```python
from build123d import *

# Parameters (mm, degrees)
BOSS_EXTRUDE2_DEPTH = 5
CHAMFER1_SIZE       = 0.7
FILLET1_R           = 2


with BuildPart() as part:
    # Sketch3 → Revolve1 (revolve)
    with BuildSketch(Plane.XY, mode=Mode.PRIVATE) as revolve1_sk:
        with BuildLine():
            Line((-41.25, 0), (-42.75, 0))
            Line((-42.75, 0), (-42.75, 15))
            Line((-42.75, 15), (-45, 15))
            add(Edge.make_bspline(
                [(-45, 15), (-45, 33.63701026), (-37.623115354, 59.484821268), (-12.301870518, 76.047426191), (0, 76.047426191)],
                knots=[0, 0, 0, 0, 0.584889903, 1, 1, 1, 1], degree=3))
            Line((0, 76.047426191), (0, 74.547426191))
            add(Edge.make_bspline(
                [(-43.490429879, 16.5), (-43.47825423, 17.447352), (-43.4296633, 19.355844405), (-43.235850844, 23.056930634), (-42.807900532, 27.545595426), (-41.986633297, 32.689505156), (-40.466663576, 39.238041503), (-37.743043327, 46.847747671), (-33.842433939, 53.728397249), (-29.961040028, 58.81673956), (-25.547541887, 63.646152056), (-20.393205683, 67.904061547), (-14.619902999, 71.183472612), (-10.010485444, 73.05966314), (-5.95200064, 74.059562605), (-2.594649158, 74.475411437), (-0.861029569, 74.547426191), (0, 74.547426191)],
                knots=[0.015975596, 0.015975596, 0.015975596, 0.015975596, 0.046726359, 0.077477122, 0.138978647, 0.200480172, 0.261981697, 0.384984748, 0.507987798, 0.569489323, 0.630990849, 0.753993899, 0.815495424, 0.87699695, 0.938498475, 0.969249237, 1, 1, 1, 1], degree=3))
            Line((-43.490429879, 16.5), (-42.75, 16.5))
            Line((-42.75, 16.5), (-41.25, 16.5))
            Line((-41.25, 16.5), (-41.25, 15))
            Line((-41.25, 15), (-41.25, 0))
        make_face()
    revolve(revolve1_sk.sketch.rotate(Axis((0, 0, 0), (0, 1, 0)), 270), axis=Axis((0, 0, 0), (0, 1, 0)))

    # Sketch4 → Boss-Extrude2 (add)
    with BuildSketch(Plane.XZ):
        with BuildLine():
            Line((-41.055602541, 4), (-4, 4))
            Line((-4, 4), (-4, 41.055602541))
            ThreePointArc((-4, 41.055602541), (0, 41.25), (4, 41.055602541))
            Line((4, 41.055602541), (4, 4))
            Line((4, 4), (41.055602541, 4))
            ThreePointArc((41.055602541, 4), (41.25, 0), (41.055602541, -4))
            Line((41.055602541, -4), (4, -4))
            Line((4, -4), (4, -41.055602541))
            ThreePointArc((4, -41.055602541), (0, -41.25), (-4, -41.055602541))
            Line((-4, -41.055602541), (-4, -4))
            Line((-4, -4), (-41.055602541, -4))
            ThreePointArc((-41.055602541, -4), (-41.25, 0), (-41.055602541, 4))
        make_face()
    extrude(amount=-BOSS_EXTRUDE2_DEPTH)

    # Chamfer1
    chamfer1_edges = [part.edges().sort_by_distance(p)[0] for p in [
        (0, 0, 42.75),
    ]]
    chamfer(chamfer1_edges, length=CHAMFER1_SIZE)

    # Fillet1
    fillet1_edges = [part.edges().sort_by_distance(p)[0] for p in [
        (-22.52780127, 5, 4),
        (-4, 5, 22.52780127),
        (4, 5, 22.52780127),
        (22.52780127, 5, 4),
        (22.52780127, 5, -4),
        (4, 5, -22.52780127),
        (-4, 5, -22.52780127),
        (-22.52780127, 5, -4),
        (-22.52780127, 0, -4),
        (-4, 0, -22.52780127),
        (4, 0, -22.52780127),
        (22.52780127, 0, -4),
        (22.52780127, 0, 4),
        (4, 0, 22.52780127),
        (-4, 0, 22.52780127),
        (-22.52780127, 0, 4),
    ]]
    fillet(fillet1_edges, radius=FILLET1_R)


solid = part.part
```
The model under review builds one solid part; all positions refer to its coordinate system, in mm. A direction names the side the tool comes from. Round coordinates to 2 decimals unless told otherwise and drop trailing zeros. Loops run counter-clockwise (first coordinate to the right, second up) from the corner with the lowest first, then second, coordinate; pieces in that order, holes last. Notation, with made-up numbers: (-25.75, 82.5) - (5.25, 82.5) arc R18 ccw to (5.25, 107.5) - close; hole circle Ø11 at (-22.75, 60). An arc over 180 degrees is marked (long way). Use a Markdown table: item, result. Add a question column.
Q1. The part is to be moulded in two halves that separate along X. For faces 1 (the face through (0, 0, -3)), 2 (the face through (-42.386, 7.95, 5.565)), 3 (the face through (0, 5, 0)), say which applies: pulls with the +X half, pulls with the -X half, needs draft (parallel to the pull), parting line crosses it, or undercut.
Q2. For probe 1 along X at (y, z) = (12, 0); probe 2 along X at (y, z) = (66.5, -12); probe 3 along Z at (x, y) = (33, 46.5), list the stretches that pass through material, from the lowest coordinate up.
Q3. Add section A-A (y = 8). State the section outline as (x, z) points, plus the area to 3 significant figures.
Q4. Insertion check: pin 1 Ø0.5 at (x, y) = (-17, 2.5) entering from -Z; pin 2 Ø0.5 at (x, y) = (-24, 2.5) entering from +Z; pin 3 Ø0.8 at (x, y) = (22.5, 2.5) entering from +Z. Each pin has a flat end and moves straight along its axis. Give the tip position at first contact, or say it passes through.
Q5. Machinability: for faces 4 (the face through (40, 15, 16)), 5 (the face through (15.9, 16.5, -38.5)), which of the approach directions +Z, -Z, +X, -X, +Y, -Y give a long, thin tool a straight path to every point of the face, cutting with its end or side? Answer none if there is none.
Worked answers:
| question | item | result |
|---|---|---|
| 1 | face 1 | needs draft |
| 1 | face 2 | parting line crosses it |
| 1 | face 3 | undercut |
| 2 | probe 1 | -42.75 to -41.25, 41.25 to 42.75 |
| 2 | probe 2 | -21.15 to -18.34, 18.34 to 21.15 |
| 2 | probe 3 | -21.23 to -18.02, 18.02 to 21.23 |
| 3 | outline | circle Ø85.5 at (0, 0); hole circle Ø82.5 at (0, 0) |
| 3 | area | 396 mm² |
| 4 | pin 1 | z = -39.33 |
| 4 | pin 2 | z = 35.55 |
| 4 | pin 3 | z = 36.59 |
| 5 | face 4 | -Y |
| 5 | face 5 | none |
